Work out the finished part from the listing and answer in its coordinate system (mm). Face numbers are marked on the shaded views. Coordinates: 2 decimals unless noted, no trailing zeros. Write each loop counter-clockwise with the first axis right and the second up, starting at its lowest first coordinate (ties: lowest second). Pieces come first, ordered by that corner, then holes. Notation, with made-up numbers: M 63,58.5 L 121,58.5 A27 ccw 121,89.5 Z; hole C 39,11 d1. An arc over 180 degrees is marked long. Use CSV: the item, a comma, the result in double quotes.
from build123d import *

# Parameters (mm, degrees)
SKETCH_2_W           = 80
SKETCH_2_H           = 34
SKETCH_2_R           = 4.05
EXTRUDE_1_DEPTH      = 8
CUT_EXTRUDE_2_DEPTH  = 88.292611371
SKETCH_5_R           = 1.55
CUT_EXTRUDE_3_DEPTH  = 88.292611371
CUT_EXTRUDE_5_DEPTH  = 4.5
SKETCH_11_R          = 1.55
CUT_EXTRUDE_7_DEPTH  = 88.292611371
CUT_EXTRUDE_11_DEPTH = 2
SKETCH_20_R          = 5.5
CUT_EXTRUDE_14_DEPTH = 88.292611371


with BuildPart() as part:
    # 草图2 → 凸台-拉伸1 (new body)
    with BuildSketch(Plane.XY):
        with Locations((40, 17)):
            Rectangle(SKETCH_2_W, SKETCH_2_H)
        with Locations((6, 8)):
            Circle(SKETCH_2_R, mode=Mode.SUBTRACT)
        with Locations((40, 10)):
            Circle(SKETCH_2_R, mode=Mode.SUBTRACT)
        with Locations((74, 8)):
            Circle(SKETCH_2_R, mode=Mode.SUBTRACT)
    extrude(amount=EXTRUDE_1_DEPTH)

    # 草图4 → 切除-拉伸2 (cut, through all)
    with BuildSketch(Plane(origin=(80, 0, 0), x_dir=(0, 0, -1), z_dir=(1, 0, 0))):
        Polygon((-1.5, 32.2), (-2.5, 32.2), (-2.5, 34), (0, 34), (0, 28.8), (-1.5, 28.8), align=None)
        Polygon((-6.5, 32.2), (-6.5, 28.8), (-8, 28.8), (-8, 34), (-5.5, 34), (-5.5, 32.2), align=None)
    extrude(amount=-CUT_EXTRUDE_2_DEPTH, mode=Mode.SUBTRACT)

    # 草图5 → 切除-拉伸3 (cut, through all)
    with BuildSketch(Plane.XY.offset(8)):
        with Locations((48, 10)):
            Circle(SKETCH_5_R)
        with Locations((32, 10)):
            Circle(SKETCH_5_R)
    extrude(amount=-CUT_EXTRUDE_3_DEPTH, mode=Mode.SUBTRACT)

    # 草图8 → 切除-拉伸5 (cut)
    with BuildSketch(Plane(origin=(0, 0, 0), x_dir=(-1, 0, 0), z_dir=(0, 0, -1))):
        Polygon((-45.15, 8.354551733), (-45.15, 11.645448267), (-48, 13.290896534), (-50.85, 11.645448267), (-50.85, 8.354551733), (-48, 6.709103466), align=None)
        Polygon((-29.15, 8.354551733), (-29.15, 11.645448267), (-32, 13.290896534), (-34.85, 11.645448267), (-34.85, 8.354551733), (-32, 6.709103466), align=None)
    extrude(amount=-CUT_EXTRUDE_5_DEPTH, mode=Mode.SUBTRACT)

    # 草图11 → 切除-拉伸7 (cut, through all)
    with BuildSketch(Plane(origin=(0, 0, 0), x_dir=(-1, 0, 0), z_dir=(0, 0, -1))):
        with Locations((-60, 25)):
            Circle(SKETCH_11_R)
        with Locations((-20, 25)):
            Circle(SKETCH_11_R)
    extrude(amount=-CUT_EXTRUDE_7_DEPTH, mode=Mode.SUBTRACT)

    # 草图19 → 切除-拉伸11 (cut)
    with BuildSketch(Plane(origin=(0, 0, 2.5), x_dir=(-1, 0, 0), z_dir=(0, 0, -1))):
        with BuildLine():
            Line((-25, 34), (-55.247938178, 34))
            Line((-55.247938178, 34), (-55.247938178, 33.2))
            ThreePointArc((-55.247938178, 33.2), (-54.747938178, 32.7), (-54.247938178, 33.2))
            Line((-54.247938178, 33.2), (-26, 33.2))
            ThreePointArc((-26, 33.2), (-25.5, 32.7), (-25, 33.2))
            Line((-25, 33.2), (-25, 34))
        make_face()
    extrude(amount=-CUT_EXTRUDE_11_DEPTH, mode=Mode.SUBTRACT)

    # 草图20 → 切除-拉伸14 (cut, through all)
    with BuildSketch(Plane(origin=(0, 0, 0), x_dir=(-1, 0, 0), z_dir=(0, 0, -1))):
        with Locations((-40, 10)):
            Circle(SKETCH_20_R)
    extrude(amount=-CUT_EXTRUDE_14_DEPTH, mode=Mode.SUBTRACT)


solid = part.part
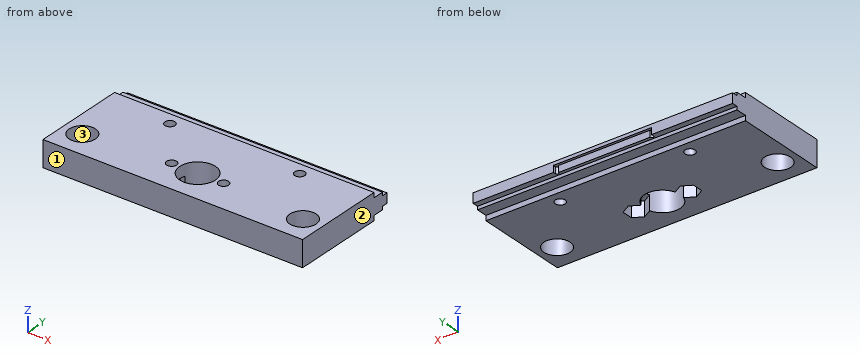
Item 1: Given pin 1 (1.4 mm diameter, centred on x = 41, y = 33.5, fed in from -Z); pin 2 (1.7 mm diameter, centred on x = 46.5, y = 30, fed in from -Z); pin 3 (3 mm diameter, centred on x = 60, y = 25, fed in from -Z); pin 4 (1.5 mm diameter, centred on x = 14.5, z = 7, fed in from +Y), each flat-ended and moving along its own axis, determine where each tip first touches the part or whether it passes through.
Answer:
pin 1,"stops at z = 2.5"
pin 2,"stops at z = 1.5"
pin 3,"passes through"
pin 4,"stops at y = 32.2"
Item 2: The part is cut by section A-A (x = 20). Write down the section's boundary in (y, z).
Answer:
outline,"M 0,0 L 23.45,0 L 23.45,8 L 0,8 Z; M 26.55,0 L 28.8,0 L 28.8,1.5 L 32.2,1.5 L 32.2,2.5 L 34,2.5 L 34,5.5 L 32.2,5.5 L 32.2,6.5 L 28.8,6.5 L 28.8,8 L 26.55,8 Z"
Item 3: For a pull along X with two mould halves and no side action, classify the marked faces 1, 2 and 3 as released by +X, released by -X, zero draft, split by the parting line, or undercut.
Answer:
face 1,"zero draft"
face 2,"released by +X"
face 3,"undercut"
Item 4: The part is cut by section D-D (x = 57.5). Write down the section's boundary in (y, z).
Answer:
outline,"M 0,0 L 28.8,0 L 28.8,1.5 L 32.2,1.5 L 32.2,2.5 L 34,2.5 L 34,5.5 L 32.2,5.5 L 32.2,6.5 L 28.8,6.5 L 28.8,8 L 0,8 Z"
Item 5: The part is cut by section C-C (y = 10). Write down the section's boundary in (x, z).
Answer:
outline,"M 0,0 L 2.48,0 L 2.48,8 L 0,8 Z; M 9.52,0 L 29.15,0 L 29.15,4.5 L 30.45,4.5 L 30.45,8 L 9.52,8 Z; M 33.55,4.5 L 34.5,4.5 L 34.5,8 L 33.55,8 Z; M 45.5,4.5 L 46.45,4.5 L 46.45,8 L 45.5,8 Z; M 49.55,4.5 L 50.85,4.5 L 50.85,0 L 70.48,0 L 70.48,8 L 49.55,8 Z; M 77.52,0 L 80,0 L 80,8 L 77.52,8 Z"
Item 6: Consider probe 1 along X at (y, z) = (10, 3.25); probe 2 along Y at (x, z) = (53.5, 6.25); probe 3 along Z at (x, y) = (34, 10). Determine where each line is inside the solid, lowest interval first.
Answer:
probe 1,"x = 0 to 2.48, 9.52 to 29.15, 50.85 to 70.48, 77.52 to 80"
probe 2,"y = 0 to 32.2"
probe 3,"z = 4.5 to 8"
Item 7: The part is cut by section B-B (y = 25). Write down the section's boundary in (x, z), then the cut area to 3 significant figures.
Answer:
outline,"M 0,0 L 18.45,0 L 18.45,8 L 0,8 Z; M 21.55,0 L 58.45,0 L 58.45,8 L 21.55,8 Z; M 61.55,0 L 80,0 L 80,8 L 61.55,8 Z"
area,"590 mm2"
